from build123d import *

# Parameters (mm, degrees)
SKETCH1_R           = 11.1125
SKETCH1_R_2         = 3.2004
EXTRUDE1_DEPTH      = 25.003125
BOSS_EXTRUDE1_START = -25.4
SKETCH8_R           = 14.2875
SKETCH8_R_2         = 3.2004
BOSS_EXTRUDE1_DEPTH = 25.4
CUT_EXTRUDE1_START  = -3.175
SKETCH5_R           = 14.2875
SKETCH5_R_2         = 3.2004
CUT_EXTRUDE1_DEPTH  = 3.175
SKETCH6_R           = 4.7625
CUT_EXTRUDE2_DEPTH  = 52.004228149
CUT_EXTRUDE3_START  = -11.77925
SKETCH7_R           = 11.1125
SKETCH7_R_2         = 8.1915
CUT_EXTRUDE3_DEPTH  = 5.334
CHAMFER2_SIZE       = 0.381
CUT_EXTRUDE4_START  = 8.9154
SKETCH9_R           = 14.2875
SKETCH9_R_2         = 11.3665
CUT_EXTRUDE4_DEPTH  = 2.667
CHAMFER3_SIZE       = 0.381
LPATTERN2_COUNT     = 3
LPATTERN2_PITCH     = 6.477


# Read off the part's stored shape, not the designer's step: LPattern1
with BuildPart() as part:
    # Sketch1 → Extrude1 (new, symmetric)
    with BuildSketch(Plane.XY):
        with Locations(Location((0, 0, 0), (0, 0, 180))):
            Circle(SKETCH1_R)
        with Locations(Location((0, 0, 0), (0, 0, 180))):
            Circle(SKETCH1_R_2, mode=Mode.SUBTRACT)
    extrude(amount=EXTRUDE1_DEPTH, both=True)

    # Sketch8 → Boss-Extrude1 (add)
    with BuildSketch(Plane.XY.offset(25.003125).offset(BOSS_EXTRUDE1_START)):
        Circle(SKETCH8_R)
        with Locations(Location((0, 0, 0), (0, 0, 180))):
            Circle(SKETCH8_R_2, mode=Mode.SUBTRACT)
    extrude(amount=BOSS_EXTRUDE1_DEPTH)

    # Sketch5 → Cut-Extrude1 (cut)
    with BuildSketch(Plane.XY.offset(25.003125).offset(CUT_EXTRUDE1_START)):
        Circle(SKETCH5_R)
        with Locations(Location((0, 0, 0), (0, 0, 180))):
            Circle(SKETCH5_R_2, mode=Mode.SUBTRACT)
    extrude(amount=CUT_EXTRUDE1_DEPTH, mode=Mode.SUBTRACT)

    # Sketch6 → Cut-Extrude2 (cut, through all)
    with BuildSketch(Plane.XY.offset(21.828125)):
        Circle(SKETCH6_R)
    extrude(amount=-CUT_EXTRUDE2_DEPTH, mode=Mode.SUBTRACT)

    # Sketch7 → Cut-Extrude3 (cut)
    with BuildSketch(Plane(origin=(0, 0, -25.003125), x_dir=(-1, 0, 0), z_dir=(0, 0, -1)).offset(CUT_EXTRUDE3_START)):
        Circle(SKETCH7_R)
        Circle(SKETCH7_R_2, mode=Mode.SUBTRACT)
    extrude(amount=CUT_EXTRUDE3_DEPTH, mode=Mode.SUBTRACT)

    # Chamfer2
    chamfer2_edges = [part.edges().sort_by_distance(p)[0] for p in [
        (11.1125, 0, -13.223875),
        (11.1125, 0, -18.557875),
    ]]
    chamfer(chamfer2_edges, length=CHAMFER2_SIZE)

    # Sketch9 → Cut-Extrude4 (cut, symmetric)
    with BuildSketch(Plane(origin=(0, 0, 21.828125), x_dir=(-1, 0, 0), z_dir=(0, 0, -1)).offset(CUT_EXTRUDE4_START)):
        with Locations(Location((0, 0, 0), (0, 0, 180))):
            Circle(SKETCH9_R)
        Circle(SKETCH9_R_2, mode=Mode.SUBTRACT)
    cut_extrude4 = extrude(amount=CUT_EXTRUDE4_DEPTH, both=True, mode=Mode.SUBTRACT)

    # Chamfer3
    chamfer3_edges = [part.edges().sort_by_distance(p)[0] for p in [
        (-14.2875, 0, 15.579725),
        (-14.2875, 0, 10.245725),
    ]]
    chamfer(chamfer3_edges, length=CHAMFER3_SIZE)

    # LPattern1 outline → LPattern1 (revolve, cut)
    with BuildSketch(Plane.XZ):
        Polygon((11.1125, -0.269875), (8.1915, -0.269875), (8.1915, -5.603875), (10.7315, -5.603875), (11.1125, -5.984875), align=None)
        Polygon((11.1125, -12.461875), (11.1125, -6.365875), (10.7315, -6.746875), (8.1915, -6.746875), (8.1915, -12.080875), (10.7315, -12.080875), align=None)
    revolve(axis=Axis((0, 0, 0), (0, 0, 1)), mode=Mode.SUBTRACT)

    # LPattern2: Cut-Extrude4 ×3
    with Locations(*[(0, 0, -i * LPATTERN2_PITCH) for i in range(1, LPATTERN2_COUNT)]):
        add(cut_extrude4, mode=Mode.SUBTRACT)


solid = part.part
The model under review builds one solid part; all positions refer to its coordinate system, in mm. A direction names the side the tool comes from. Round coordinates to 2 decimals unless told otherwise and drop trailing zeros. Loops run counter-clockwise (first coordinate to the right, second up) from the corner with the lowest first, then second, coordinate; pieces in that order, holes last. Notation, with made-up numbers: M 7.25,-32 L 62.25,-32 A19 cw 62.25,-25 Z; hole C 47,61.5 d1. An arc over 180 degrees is marked long. Answer as CSV lines item,"result". Start each with the question number.
Item 1: Insertion check: P1, Ø12, axis at y = -8.5, z = -5.5, coming from the +X side; P2, Ø6, axis at x = 0, z = -16.5, coming from the -Y side; P3, Ø1.5, axis at x = -6, z = -20, coming from the -Y side. Each pin has a flat end and moves straight along its axis. Give the tip position at first contact, or say it passes through.
Item 2: Mouldability with a two-part tool opening along Y and no side actions: class faces 1 (the face through (-3.78, -2.9, -1.26)), 2 (the face through (2.464, -11.096, 1.136)), 3 (the face through (-10, 6, 9.103)) as released by +Y, released by -Y, zero draft, split by the parting line, or undercut.
Item 3: Consider section C-C (z = -10). Write out the cut boundary in (x, y) (1 decimal).
Item 4: Consider section A-A (z = 6). Write out the cut boundary in (x, y) (1 decimal), then the cut area to 3 significant figures.
Item 5: Consider section B-B (y = -9). State how many separate pieces and enclosed holes the cut face has, then the cut area to 3 significant figures.
Item 6: For faces 4 (the face through (8.2, -7.5, -21.9)), 5 (the face through (0, 5, -25.003)), 6 (the face through (-3, -8, -18.558)), list the 3-axis set-ups (+Z, -Z, +X, -X, +Y, -Y) from which the entire face can be reached by the end or side of a thin tool; tool diameter is ignored.
Item 7: Wall thickness on line 1 (Z direction, x = -7.5, y = -10); line 2 (Z direction, x = 6.25, y = -7); line 3 (Y direction, x = 0, z = -0.3): over which ranges is each line inside the solid? List them lowest first. Write a range as [from, to].
Answer:
1,P1,"stops at x = 10.82"
1,P2,"stops at y = -11.11"
1,P3,"stops at y = -9.79"
2,face 1,"undercut"
2,face 2,"split by the parting line"
2,face 3,"zero draft"
3,outline,"C 0,0 d16.4; hole C 0,0 d9.5"
4,outline,"C 0,0 d22.7; hole C 0,0 d9.5"
4,area,"335 mm^2"
5,separate pieces,"4"
5,enclosed holes,"0"
5,area,"490 mm^2"
6,face 4,"-Z"
6,face 5,"-Z, +X, -X, +Y, -Y"
6,face 6,"none"
7,line 1,"z = [2.63, 3.77], [9.1, 10.25], [15.58, 21.83]"
7,line 2,"z = [-25, -18.56], [-13.22, -12.08], [-6.75, -5.6], [-0.27, 21.83]"
7,line 3,"y = [-11.37, -11.11], [-8.19, -4.76], [4.76, 8.19], [11.11, 11.37]"
